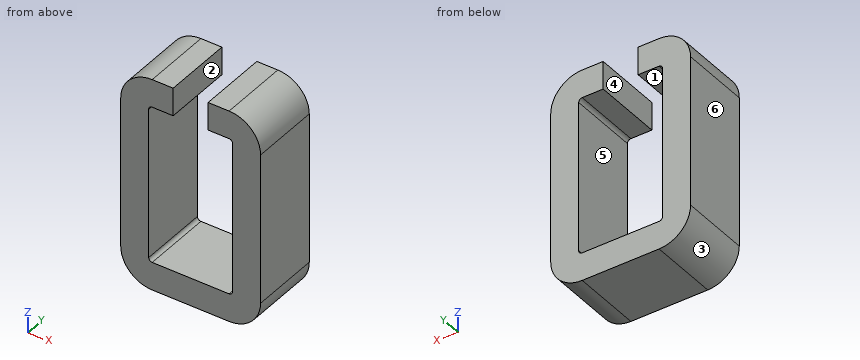
```python
from build123d import *

# Parameters (mm, degrees)
BOSS_EXTRUDE1_DEPTH = 10


with BuildPart() as part:
    # Sketch1 → Boss-Extrude1 (new body)
    with BuildSketch(Plane(origin=(0, 0, 0), x_dir=(1, 0, 0), z_dir=(0, 1, 0))):
        with BuildLine():
            Line((-4, -0.5), (-4, -22))
            ThreePointArc((-4, -22), (-2.681980515, -25.181980515), (0.5, -26.5))
            Line((0.5, -26.5), (3.5, -26.5))
            Line((3.5, -26.5), (3.5, -22.5))
            Line((3.5, -22.5), (0.5, -22.5))
            ThreePointArc((0.5, -22.5), (0.146446609, -22.353553391), (0, -22))
            Line((0, -22), (0, -0.5))
            ThreePointArc((0, -0.5), (0.146446609, -0.146446609), (0.5, 0))
            Line((0.5, 0), (11.5, 0))
            ThreePointArc((11.5, 0), (11.853553391, -0.146446609), (12, -0.5))
            Line((12, -0.5), (12, -22))
            ThreePointArc((12, -22), (11.853553391, -22.353553391), (11.5, -22.5))
            Line((11.5, -22.5), (8.5, -22.5))
            Line((8.5, -22.5), (8.5, -26.5))
            Line((8.5, -26.5), (11.5, -26.5))
            ThreePointArc((11.5, -26.5), (14.681980515, -25.181980515), (16, -22))
            Line((16, -22), (16, -0.5))
            ThreePointArc((16, -0.5), (14.681980515, 2.681980515), (11.5, 4))
            Line((11.5, 4), (0.5, 4))
            ThreePointArc((0.5, 4), (-2.681980515, 2.681980515), (-4, -0.5))
        make_face()
    extrude(amount=BOSS_EXTRUDE1_DEPTH)


solid = part.part
```
Geometry: final body of the model. Coordinates: model frame, mm. Face numbers are marked on the shaded views. A direction names the side the tool comes from. Round coordinates to 2 decimals unless told otherwise and drop trailing zeros. Loops run counter-clockwise (first coordinate to the right, second up) from the corner with the lowest first, then second, coordinate; pieces in that order, holes last. Notation, with made-up numbers: (53, 65) -> (75, 65) arc R15 cw to (75, 87) -> close; hole circle Ø4 at (-30.75, 63). An arc over 180 degrees is marked (long way). Use one line per item in the form item = value. Start each with the question number.
1) Section C-C on y = 7.25. Output: boundary loops of the cut face in (x, z), then the cut area to 3 significant figures.
2) First-contact query: P1, Ø1, axis at x = -1, y = 6, coming from the -Z side; P2, Ø1.2, axis at y = 7, z = 24.5, coming from the -X side; P3, Ø1.2, axis at y = 2.5, z = 24.5, coming from the +X side. Flat tips, straight axial feed; report the tip coordinate or a pass-through.
3) Draft query along Z for the marked faces 1, 2 and 3. Return one class per face: released by +Z, released by -Z, zero draft, split by the parting line, or undercut.
4) Line query: L1, parallel to X at y = 4.5, z = 4; L2, parallel to Z at x = 0.75, y = 3.25; L3, parallel to Z at x = 6, y = 3.75. Output: solid intervals per line, ascending.
5) Access query for the marked faces 4, 5 and 6. Directions: +Z, -Z, +X, -X, +Y, -Y. A direction counts if a zero-diameter tool reaches every point of the face in a straight line with its end or side. Return the directions, or none.
6) Section D-D on z = -1. Output: boundary loops of the cut face in (x, y), then the cut area to 3 significant figures.
7) Section B-B on x = 11. Output: boundary loops of the cut face in (y, z), then the cut area to 3 significant figures.
8) Section A-A on z = 19. Output: boundary loops of the cut face in (x, y), then the cut area to 3 significant figures.
Response:
q1.outline = (-4, 0.5) arc R4.5 ccw to (0.5, -4) -> (11.5, -4) arc R4.5 ccw to (16, 0.5) -> (16, 22) arc R4.5 ccw to (11.5, 26.5) -> (8.5, 26.5) -> (8.5, 22.5) -> (11.5, 22.5) arc R0.5 cw to (12, 22) -> (12, 0.5) arc R0.5 cw to (11.5, 0) -> (0.5, 0) arc R0.5 cw to (0, 0.5) -> (0, 22) arc R0.5 cw to (0.5, 22.5) -> (3.5, 22.5) -> (3.5, 26.5) -> (0.5, 26.5) arc R4.5 ccw to (-4, 22) -> close
q1.area = 303 mm^2
q2.P1 = -3.89
q2.P2 = -3.58
q2.P3 = 15.58
q3.face_1 = undercut
q3.face_2 = zero draft
q3.face_3 = released by -Z
q4.L1 = -4 to 0, 12 to 16
q4.L2 = -4 to 0, 22.5 to 26.5
q4.L3 = -4 to 0
q5.face_4 = +Z, +Y, -Y
q5.face_5 = +Y, -Y
q5.face_6 = +Z, -Z, -X, +Y, -Y
q6.outline = (-3.74, 0) -> (15.74, 0) -> (15.74, 10) -> (-3.74, 10) -> close
q6.area = 195 mm^2
q7.outline = (0, -4) -> (10, -4) -> (10, 0) -> (0, 0) -> close; (0, 22.5) -> (10, 22.5) -> (10, 26.5) -> (0, 26.5) -> close
q7.area = 80.0 mm^2
q8.outline = (-4, 0) -> (0, 0) -> (0, 10) -> (-4, 10) -> close; (12, 0) -> (16, 0) -> (16, 10) -> (12, 10) -> close
q8.area = 80.0 mm^2
